```python
from build123d import *

# Parameters (mm, degrees)
SKETCH_W        = 30
SKETCH_H        = 30
PAD_DEPTH       = 15
SKETCH001_W     = 26
SKETCH001_H     = 26
POCKET_DEPTH    = 13
SKETCH002_W     = 5.5
SKETCH002_H     = 26
PAD001_DEPTH    = 5
SKETCH003_W     = 20
SKETCH003_H     = 4
POCKET001_DEPTH = 5
SKETCH004_R     = 4
POCKET002_DEPTH = 5
SKETCH005_W     = 5
SKETCH005_H     = 15
PAD002_DEPTH    = 15
SKETCH006_R     = 1.6
POCKET003_DEPTH = 30.001
FILLET_R        = 3
FILLET001_R     = 3
FILLET002_R     = 1


with BuildPart() as part:
    # Sketch → Pad (new body)
    with BuildSketch(Plane.XY):
        with Locations((-15, 15)):
            Rectangle(SKETCH_W, SKETCH_H)
    extrude(amount=PAD_DEPTH)

    # Sketch001 (on Face6 of Pad) → Pocket (cut)
    with BuildSketch(Plane.XY.offset(15)):
        with Locations((-15, 15)):
            Rectangle(SKETCH001_W, SKETCH001_H)
    extrude(amount=-POCKET_DEPTH, mode=Mode.SUBTRACT)

    # Sketch002 (on Face11 of Pocket) → Pad001 (join)
    with BuildSketch(Plane.XY.offset(2)):
        with Locations((-25.25, 15)):
            Rectangle(SKETCH002_W, SKETCH002_H)
        with Locations((-4.75, 15)):
            Rectangle(SKETCH002_W, SKETCH002_H)
    extrude(amount=PAD001_DEPTH)

    # Sketch003 (on Face9 of Pad001) → Pocket001 (cut)
    with BuildSketch(Plane(origin=(0, 2, 0), x_dir=(-1, 0, 0), z_dir=(0, 1, 0))):
        with Locations((15, 9)):
            Rectangle(SKETCH003_W, SKETCH003_H)
    extrude(amount=-POCKET001_DEPTH, mode=Mode.SUBTRACT)

    # Sketch004 (on Face19 of Pocket001) → Pocket002 (cut)
    with BuildSketch(Plane.XY.offset(2)):
        with Locations((-15, 12.5)):
            Circle(SKETCH004_R)
    extrude(amount=-POCKET002_DEPTH, mode=Mode.SUBTRACT)

    # Sketch005 (on Face1 of Pocket002) → Pad002 (join)
    with BuildSketch(Plane.XZ):
        with Locations((-27.5, 7.5)):
            Rectangle(SKETCH005_W, SKETCH005_H)
        with Locations((-2.5, 7.5)):
            Rectangle(SKETCH005_W, SKETCH005_H)
    extrude(amount=PAD002_DEPTH)

    # Sketch006 (on Face22 of Pad002) → Pocket003 (cut, through all)
    with BuildSketch(Plane.YZ):
        with Locations((-10.757359, 4.242641)):
            Circle(SKETCH006_R)
        with BuildLine():
            ThreePointArc((0, 15), (-8.276473, 13.16387), (-15, 8))
            Line((-15, 8), (-15, 15))
            Line((-15, 15), (0, 15))
        make_face()
    extrude(amount=-POCKET003_DEPTH, mode=Mode.SUBTRACT)

    # Fillet
    fillet_edges = [part.edges().sort_by_distance(p)[0] for p in [
        (-30, 30, 7.5),
        (0, 30, 7.5),
    ]]
    fillet(fillet_edges, radius=FILLET_R)

    # Fillet001
    fillet001_edges = [part.edges().sort_by_distance(p)[0] for p in [
        (-30, -15, 4),
        (0, -15, 4),
    ]]
    fillet(fillet001_edges, radius=FILLET001_R)

    # Fillet002
    fillet002_edges = [part.edges().sort_by_distance(p)[0] for p in [
        (-19, 12.5, 0),
    ]]
    fillet(fillet002_edges, radius=FILLET002_R)


solid = part.part
```
Build history of the part. All positions in model axes, mm. A direction names the side the tool comes from. Round coordinates to 2 decimals unless told otherwise and drop trailing zeros. Write each loop counter-clockwise with the first axis right and the second up, starting at its lowest first coordinate (ties: lowest second). Pieces come first, ordered by that corner, then holes. Notation, with made-up numbers: (67.25, 11.25) -> (120.25, 11.25) arc R35 cw to (120.25, 49.25) -> close; hole circle Ø5 at (72.25, 30.25). An arc over 180 degrees is marked (long way). Put each result on its own line as item: value.
Item 1: Slice it at B-B, the plane x = -15. Give the cut face in (y, z), plus the area to 3 significant figures.
Here are the results:
outline: (0, 0) -> (7.5, 0) arc R1 ccw to (8.5, 1) -> (8.5, 2) -> (2, 2) -> (2, 7) -> (0, 7) -> close; (0, 11) -> (2, 11) -> (2, 15) -> (0, 15) -> close; (16.5, 1) arc R1 ccw to (17.5, 0) -> (30, 0) -> (30, 15) -> (28, 15) -> (28, 2) -> (16.5, 2) -> close
area: 87.6 mm^2
Item 2: Slice it at A-A, the plane y = 12.5. Give the cut face in (x, z), plus the area to 3 significant figures.
Here are the results:
outline: (-30, 0) -> (-20, 0) arc R1 ccw to (-19, 1) -> (-19, 2) -> (-22.5, 2) -> (-22.5, 7) -> (-28, 7) -> (-28, 15) -> (-30, 15) -> close; (-11, 1) arc R1 ccw to (-10, 0) -> (0, 0) -> (0, 15) -> (-2, 15) -> (-2, 7) -> (-7.5, 7) -> (-7.5, 2) -> (-11, 2) -> close
area: 151 mm^2
Item 3: Flat gauge pins, fed straight in: P1, Ø1.5, axis at x = -16, y = 16, coming from the -Z side; P2, Ø12, axis at x = -12.5, y = 9, coming from the +Z side; P3, Ø1.5, axis at x = -11.5, z = 9, coming from the -Y side. Where does each tip first touch, or does it go through?
Here are the results:
P1: stops at z = 0.21
P2: stops at z = 7
P3: stops at y = 28
Item 4: Wall check: probe 1 along X at (y, z) = (-5.5, 8); probe 2 along Y at (x, z) = (-15, 1.8); probe 3 along X at (y, z) = (7, 10.5). Give the ranges that are in metal, low to high. Write a range as from..to.
Here are the results:
probe 1: x = -30..-25, -5..0
probe 2: y = 0..8.5, 16.5..30
probe 3: x = -30..-28, -2..0
Item 5: Tool access for faces 4 (the face through (-15, 0, 3)), 5 (the face through (-15, 1, 11)), 6 (the face through (-2, 15, 11)): list every direction of +Z, -Z, +X, -X, +Y, -Y with a clear straight run to the whole face (end or side of a thin tool).
Here are the results:
face 4: +Z, -Z, -Y
face 5: -Y
face 6: +Z
Item 6: Two-plate mould, pull along X, no slides. Class faces 1 (the face through (-27.465, -9.897, 5.592)), 2 (the face through (0, 7, 7)), 3 (the face through (-22.5, 15, 4)): pulls with the +X half, pulls with the -X half, needs draft (parallel to the pull), parting line crosses it, or undercut.
Here are the results:
face 1: needs draft
face 2: pulls with the +X half
face 3: undercut
Item 7: Slice it at C-C, the plane z = 7.5. Give the cut face in (x, y).
Here are the results:
outline: (-30, -12) arc R3 ccw to (-27, -15) -> (-25, -15) -> (-25, 2) -> (-28, 2) -> (-28, 28) -> (-2, 28) -> (-2, 2) -> (-5, 2) -> (-5, -15) -> (-3, -15) arc R3 ccw to (0, -12) -> (0, 27) arc R3 ccw to (-3, 30) -> (-27, 30) arc R3 ccw to (-30, 27) -> close
Item 8: Slice it at D-D, the plane x = -4.5. Give the cut face in (y, z), plus the area to 3 significant figures.
Here are the results:
outline: (-15, 0) -> (30, 0) -> (30, 15) -> (28, 15) -> (28, 7) -> (2, 7) -> (2, 15) -> (0, 15) arc R19.57 ccw to (-15, 8) -> close; hole circle Ø3.2 at (-10.76, 4.24)
area: 427 mm^2
